For this review, take the finished solid that the model builds, in its own axes (mm). A direction names the side the tool comes from. Give positions to 0.01 mm unless a question says otherwise; leave off trailing zeros. Write each loop counter-clockwise with the first axis right and the second up, starting at its lowest first coordinate (ties: lowest second). Pieces come first, ordered by that corner, then holes. Notation, with made-up numbers: (-25, 39.5) -> (4, 39.5) arc R22 ccw to (4, 70.5) -> close; hole circle Ø3 at (50.25, 79). An arc over 180 degrees is marked (long way). Return JSON: item names as keys, results as strings.
from build123d import *

# Parameters (mm, degrees)
SKETCH1_R           = 4.7625
SKETCH1_R_2         = 4.0513
BOSS_EXTRUDE1_DEPTH = 127
SKETCH2_R           = 3.175
CUT_EXTRUDE1_DEPTH  = 5.7625


with BuildPart() as part:
    # Sketch1 → Boss-Extrude1 (new body, symmetric)
    with BuildSketch(Plane(origin=(0, 0, 0), x_dir=(0, 0, -1), z_dir=(1, 0, 0))):
        Circle(SKETCH1_R)
        Circle(SKETCH1_R_2, mode=Mode.SUBTRACT)
    extrude(amount=BOSS_EXTRUDE1_DEPTH, both=True)

    # Sketch2 → Cut-Extrude1 (cut, through all)
    with BuildSketch(Plane(origin=(0, 0, 0), x_dir=(1, 0, 0), z_dir=(0, 1, 0))):
        with Locations((-112.5, 0)):
            Circle(SKETCH2_R)
        with Locations((-37.5, 0)):
            Circle(SKETCH2_R)
        with Locations((37.5, 0)):
            Circle(SKETCH2_R)
        with Locations((112.5, 0)):
            Circle(SKETCH2_R)
    extrude(amount=-CUT_EXTRUDE1_DEPTH, mode=Mode.SUBTRACT)


solid = part.part
1. Add section A-A, the plane z = 0. State the section outline as (x, y) points (1 decimal).
Results found:
{"outline": "(-127, -4.8) -> (-115.7, -4.8) -> (-115.7, -4.1) -> (-127, -4.1) -> close; (-127, 4.1) -> (127, 4.1) -> (127, 4.8) -> (-127, 4.8) -> close; (-109.3, -4.8) -> (-40.7, -4.8) -> (-40.7, -4.1) -> (-109.3, -4.1) -> close; (-34.3, -4.8) -> (34.3, -4.8) -> (34.3, -4.1) -> (-34.3, -4.1) -> close; (40.7, -4.8) -> (109.3, -4.8) -> (109.3, -4.1) -> (40.7, -4.1) -> close; (115.7, -4.8) -> (127, -4.8) -> (127, -4.1) -> (115.7, -4.1) -> close"}
2. To check wall thickness, follow probe 1 along X at (y, z) = (-4.1, 0) (3 decimals); probe 2 along Y at (x, z) = (85, 0.5); probe 3 along Y at (x, z) = (52.5, 0). State the ranges of each line that lie inside material, in increasing order.
Results found:
{"probe 1": "x = -127 to -115.675, -109.325 to -40.675, -34.325 to 34.325, 40.675 to 109.325, 115.675 to 127", "probe 2": "y = -4.74 to -4.02, 4.02 to 4.74", "probe 3": "y = -4.76 to -4.05, 4.05 to 4.76"}
3. Add section D-D, the plane x = 37.5. State the section outline as (y, z) points (1 decimal), plus the area to 3 significant figures.
Results found:
{"outline": "(-3.5, -3.2) arc R4.8 ccw (long way) to (-3.5, 3.2) -> (-2.5, 3.2) arc R4.1 cw (long way) to (-2.5, -3.2) -> close", "area": "14.6 mm²"}
4. For faces 1 (the cylindrical face through (39.207, -3.628, -2.677)), 2 (the flat face through (-127, 4, -2)), list the 3-axis set-ups (+Z, -Z, +X, -X, +Y, -Y) from which the entire face can be reached by the end or side of a thin tool; tool diameter is ignored.
Results found:
{"face 1": "-Y", "face 2": "+Z, -Z, -X, +Y, -Y"}
5. The part is to be moulded in two halves that separate along Z. For faces 3 (the flat face through (127, 4, -2)), 4 (the cylindrical face through (114.207, -3.628, -2.677)), 5 (the cylindrical face through (1.78, 4.72, 0.62)), say which applies: +Z half, -Z half, draft (parallel to the pull), parting line (faces both ways), or undercut.
Results found:
{"face 3": "draft", "face 4": "undercut", "face 5": "parting line"}
6. Add section B-B, the plane y = 0. State the section outline as (x, z) points, plus the area to 3 significant figures.
Results found:
{"outline": "(-127, -4.76) -> (127, -4.76) -> (127, -4.05) -> (-127, -4.05) -> close; (-127, 4.05) -> (127, 4.05) -> (127, 4.76) -> (-127, 4.76) -> close", "area": "361 mm²"}
7. Add section C-C, the plane x = -50. State the section outline as (y, z) points (1 decimal).
Results found:
{"outline": "circle Ø9.5 at (0, 0); hole circle Ø8.1 at (0, 0)"}
8. For pin 1 (1.5 mm diameter, centred on x = -27, z = 1, fed in from -Y); pin 2 (5 mm diameter, centred on x = -37.5, z = 0, fed in from -Y), all flat-tipped, find the tip position at first contact; note any pin that passes through.
Results found:
{"pin 1": "stops at y = -4.76", "pin 2": "stops at y = 3.19"}
